```python
from build123d import *

# Parameters (mm, degrees)
F0_W     = 101.6
F0_H     = 27.94
F1_DEPTH = 5.08
F3_D     = 6.35
F5_D     = 12.7


with BuildPart() as f1:
    # F0 (on Front) → F1 (new body)
    with BuildSketch(Plane.XZ):
        Rectangle(F0_W, F0_H)
    extrude(amount=F1_DEPTH)

    # F3 (through all)
    with Locations(Plane.XZ.offset(5.08)):
        with Locations((-38.1, 0), (38.1, 0)):
            Hole(F3_D / 2)

    # F5 (through all)
    with Locations(Plane.XZ.offset(5.08)):
        with Locations((0, 0)):
            Hole(F5_D / 2)


solid = f1.part
```
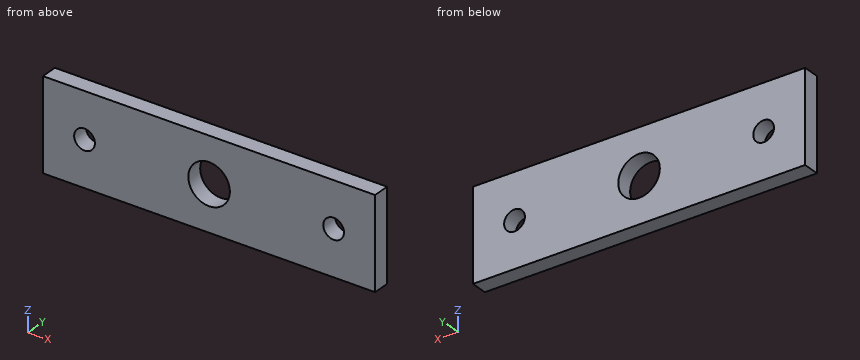
Could you check a few things on this model? Use its own coordinates, in mm. Coordinates: 2 decimals unless noted, no trailing zeros. Loops run counter-clockwise (first coordinate to the right, second up) from the corner with the lowest first, then second, coordinate; pieces in that order, holes last. Notation, with made-up numbers: M 12,-12 L 62,-12 A19 cw 62,1 Z; hole C 56.5,77 d2. An arc over 180 degrees is marked long. Put each result on its own line as item: value. Start each with the question number.
(1) I need wall thicknesses on line 1 (Z direction, x = 38.1, y = -2.5) (3 decimals); line 2 (Z direction, x = 0, y = -1.6); line 3 (X direction, y = -3.05, z = 1). Which ranges of each line are inside material? Lowest first, please. Write a range as from..to.
(2) Suppose I cut it at A-A on x = 0. Please give me the cut outline in (y, z).
(3) Suppose I cut it at C-C on y = -2.3. Please give me the cut outline in (x, z) (3 decimals).
(4) Suppose I cut it at D-D on x = 38.1. Please give me the cut outline in (y, z) (3 decimals).
(5) Suppose I cut it at B-B on z = 0. Please give me the cut outline in (x, y) (3 decimals).
Solutions:
1. line 1: z = -13.97..-3.175, 3.175..13.97
1. line 2: z = -13.97..-6.35, 6.35..13.97
1. line 3: x = -50.8..-41.11, -35.09..-6.27, 6.27..35.09, 41.11..50.8
2. outline: M -5.08,-13.97 L 0,-13.97 L 0,-6.35 L -5.08,-6.35 Z; M -5.08,6.35 L 0,6.35 L 0,13.97 L -5.08,13.97 Z
3. outline: M -50.8,-13.97 L 50.8,-13.97 L 50.8,13.97 L -50.8,13.97 Z; hole C -38.1,0 d6.35; hole C 0,0 d12.7; hole C 38.1,0 d6.35
4. outline: M -5.08,-13.97 L 0,-13.97 L 0,-3.175 L -5.08,-3.175 Z; M -5.08,3.175 L 0,3.175 L 0,13.97 L -5.08,13.97 Z
5. outline: M -50.8,-5.08 L -41.275,-5.08 L -41.275,0 L -50.8,0 Z; M -34.925,-5.08 L -6.35,-5.08 L -6.35,0 L -34.925,0 Z; M 6.35,-5.08 L 34.925,-5.08 L 34.925,0 L 6.35,0 Z; M 41.275,-5.08 L 50.8,-5.08 L 50.8,0 L 41.275,0 Z
